```python
from build123d import *

# Parameters (mm, degrees)
CROQUIS1_R              = 2.5
SALIENTE_EXTRUIR1_DEPTH = 3


with BuildPart() as part:
    # Croquis1 → Saliente-Extruir1 (new body)
    with BuildSketch(Plane.XY):
        with BuildLine():
            Line((20, 0), (20, 83))
            ThreePointArc((20, 83), (19.414213562, 84.414213562), (18, 85))
            Line((18, 85), (2, 85))
            ThreePointArc((2, 85), (0.585786438, 84.414213562), (0, 83))
            Line((0, 83), (0, 0))
            Line((0, 0), (20, 0))
        make_face()
        with Locations((10, 76.69)):
            Circle(CROQUIS1_R, mode=Mode.SUBTRACT)
        with Locations((10, 40.69)):
            Circle(CROQUIS1_R, mode=Mode.SUBTRACT)
    extrude(amount=SALIENTE_EXTRUIR1_DEPTH)


solid = part.part
```
Design review of the part built by this model. Coordinates are the model's own, in mm. Round coordinates to 2 decimals unless told otherwise and drop trailing zeros. Write each loop counter-clockwise with the first axis right and the second up, starting at its lowest first coordinate (ties: lowest second). Pieces come first, ordered by that corner, then holes. Notation, with made-up numbers: (1.5, 36.5) -> (53.5, 36.5) arc R18 ccw to (53.5, 57.5) -> close; hole circle Ø2 at (-10.75, 74.5). An arc over 180 degrees is marked (long way). Answer in a Markdown table with one row per item.
Q1. Take a section at A-A, the plane z = 1.9. State the section outline as (x, y) points.
The answers:
| item | result |
|---|---|
| outline | (0, 0) -> (20, 0) -> (20, 83) arc R2 ccw to (18, 85) -> (2, 85) arc R2 ccw to (0, 83) -> close; hole circle Ø5 at (10, 40.69); hole circle Ø5 at (10, 76.69) |
Q2. Draft analysis for pull direction Y (two halves, no side actions). For faces 1 (the face through (0.6, 84.43, 1.48)), 2 (the face through (10, 0, 1)), 3 (the face through (11.34, 42.8, 1.48)), state which applies: +Y half, -Y half, draft (parallel to the pull), parting line (faces both ways), or undercut.
The answers:
| item | result |
|---|---|
| face 1 | +Y half |
| face 2 | -Y half |
| face 3 | undercut |
Q3. To check wall thickness, follow L1, parallel to Y at x = 10, z = 1.6; L2, parallel to Y at x = 18.25, z = 0.65; L3, parallel to Y at x = 18.5, z = 0.5. State the ranges of each line that lie inside material, in increasing order. Write a range as [from, to].
The answers:
| item | result |
|---|---|
| L1 | [0, 38.19], [43.19, 74.19], [79.19, 85] |
| L2 | [0, 84.98] |
| L3 | [0, 84.94] |
Q4. Take a section at B-B, the plane x = 10. State the section outline as (y, z) points.
The answers:
| item | result |
|---|---|
| outline | (0, 0) -> (38.19, 0) -> (38.19, 3) -> (0, 3) -> close; (43.19, 0) -> (74.19, 0) -> (74.19, 3) -> (43.19, 3) -> close; (79.19, 0) -> (85, 0) -> (85, 3) -> (79.19, 3) -> close |
Q5. Take a section at C-C, the plane y = 76.69. State the section outline as (x, z) points.
The answers:
| item | result |
|---|---|
| outline | (0, 0) -> (7.5, 0) -> (7.5, 3) -> (0, 3) -> close; (12.5, 0) -> (20, 0) -> (20, 3) -> (12.5, 3) -> close |
